Source: CAD feature listing. Evaluate the final solid. Frame: model axes, mm. Face numbers are marked on the shaded views. A direction names the side the tool comes from. Round coordinates to 2 decimals unless told otherwise and drop trailing zeros. Order: outer loops, then holes, each group sorted by start corner. A loop starts at its lowest first (then second) coordinate and runs counter-clockwise, first axis right, second up. Notation, with made-up numbers: (-28.75, 59.5) -> (21.25, 59.5) arc R32 cw to (21.25, 90.5) -> close; hole circle Ø9 at (61.5, -12). An arc over 180 degrees is marked (long way). Write item = value, one per line. Start each with the question number.
(1) Cut plane C-C on z = 11. Return the cut outline in (x, y), then the cut area to 3 significant figures.
(2) Cut plane D-D on x = -8. Return the cut outline in (y, z) (3 decimals), then the cut area to 3 significant figures.
(3) Cut plane A-A on z = 1.5. Return the cut outline in (x, y), then the cut area to 3 significant figures.
(4) Reachability of the marked faces 4, 5 and 6 from +Z, -Z, +X, -X, +Y, -Y: full face, straight path, thin tool, end or side. Return the list, or none.
(5) Contact query for flat-ended pins moving along their axis: pin 1 Ø5 at (y, z) = (1.5, 11) entering from +X; pin 2 Ø1.9 at (y, z) = (8, 21) entering from -X; pin 3 Ø10 at (x, y) = (-2, 6) entering from +Z (3 decimals); pin 4 Ø7 at (y, z) = (8, 19.6) entering from -X. Output: stop coordinate, or through.
(6) Ray query, line 1 (Y direction, x = 11.7, z = 19.6); line 2 (Y direction, x = 7, z = 19.25); line 3 (Z direction, x = 9, y = -1.75) (3 decimals). Return the intervals inside material, ascending.
(7) Draft query along X for the marked faces 1, 2 and 3. Return one class per face: released by +X, released by -X, zero draft, split by the parting line, or undercut.
(8) Cut plane B-B on y = 9.75. Return the cut outline in (x, z) (3 decimals).
from build123d import *

# Parameters (mm, degrees)
BOSS_EXTRUDE1_DEPTH   = 11.5
SKETCH3_R             = 2.4
CUT_EXTRUDE1_DEPTH    = 38.4
SKETCH3_3_R           = 3.1
SKETCH3_3_R_2         = 2.4
CUT_EXTRUDE2_DEPTH    = 0.8
FILLET1_R             = 3.6
F_8_CLEARANCE_HOLE1_D = 4.4958


with BuildPart() as part:
    # Sketch2 → Boss-Extrude1 (new body, symmetric)
    with BuildSketch(Plane(origin=(0, 0, 0), x_dir=(1, 0, 0), z_dir=(0, 1, 0))):
        Polygon((4, -3.175), (4, -19.599999916), (4, -23.199999916), (12, -23.199999916), (12, -19.599999916), (12, -3.175), (25.4, -3.175), (25.4, 3.175), (-25.4, 3.175), (-25.4, -3.175), align=None)
    extrude(amount=BOSS_EXTRUDE1_DEPTH, both=True)

    # Sketch3 → Cut-Extrude1 (cut, through all)
    with BuildSketch(Plane(origin=(12, 0, 0), x_dir=(0, 0, -1), z_dir=(1, 0, 0))):
        with Locations((-19.599999916, 8)):
            Circle(SKETCH3_R)
        with BuildLine():
            ThreePointArc((-17.337258216, 0.73137085), (-17.232272581, 0), (-17.337258216, -0.73137085))
            Line((-17.337258216, -0.73137085), (-18.799999916, -0.73137085))
            Line((-18.799999916, -0.73137085), (-18.799999916, -2.19411255))
            ThreePointArc((-18.799999916, -2.19411255), (-19.599999916, -2.320249175), (-20.399999916, -2.19411255))
            Line((-20.399999916, -2.19411255), (-20.399999916, -0.73137085))
            Line((-20.399999916, -0.73137085), (-21.862741616, -0.73137085))
            ThreePointArc((-21.862741616, -0.73137085), (-21.967727251, 0), (-21.862741616, 0.73137085))
            Line((-21.862741616, 0.73137085), (-20.399999916, 0.73137085))
            Line((-20.399999916, 0.73137085), (-20.399999916, 2.19411255))
            ThreePointArc((-20.399999916, 2.19411255), (-19.599999916, 2.320249175), (-18.799999916, 2.19411255))
            Line((-18.799999916, 2.19411255), (-18.799999916, 0.73137085))
            Line((-18.799999916, 0.73137085), (-17.337258216, 0.73137085))
        make_face()
        with Locations((-19.599999916, -8)):
            Circle(SKETCH3_R)
    extrude(amount=-CUT_EXTRUDE1_DEPTH, mode=Mode.SUBTRACT)

    # Sketch3_3 → Cut-Extrude2 (cut)
    with BuildSketch(Plane(origin=(12, 0, 0), x_dir=(0, 0, -1), z_dir=(1, 0, 0))):
        with Locations((-19.599999916, 8)):
            Circle(SKETCH3_3_R)
        with Locations((-19.599999916, 8)):
            Circle(SKETCH3_3_R_2, mode=Mode.SUBTRACT)
        with Locations((-19.599999916, -8)):
            Circle(SKETCH3_3_R)
        with Locations((-19.599999916, -8)):
            Circle(SKETCH3_3_R_2, mode=Mode.SUBTRACT)
    cut_extrude2 = extrude(amount=-CUT_EXTRUDE2_DEPTH, mode=Mode.SUBTRACT)

    # Mirror1: Cut-Extrude2 across plane
    add(cut_extrude2.mirror(Plane(origin=(8, 0, 0), x_dir=(0, 0, 1), z_dir=(1, 0, 0))), mode=Mode.SUBTRACT)

    # Fillet1
    fillet1_edges = [part.edges().sort_by_distance(p)[0] for p in [
        (8, -11.5, 23.199999916),
        (12, 0, 3.175),
        (4, 0, 3.175),
        (8, 11.5, 23.199999916),
    ]]
    fillet(fillet1_edges, radius=FILLET1_R)

    # 8 Clearance Hole1 (through all)
    with Locations(Plane.XY.offset(3.175)):
        with Locations((-20.6375, 6.7375), (-20.6375, -6.7375), (20.6375, -6.7375), (20.6375, 6.7375)):
            Hole(F_8_CLEARANCE_HOLE1_D / 2)


solid = part.part
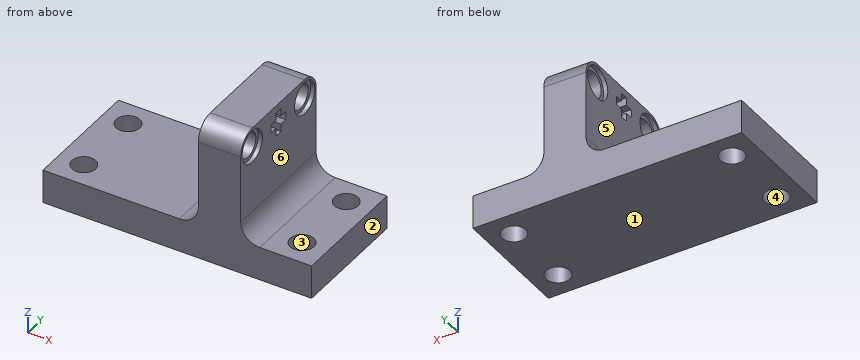
Evaluation:
q1.outline = (4, -11.5) -> (12, -11.5) -> (12, 11.5) -> (4, 11.5) -> close
q1.area = 184 mm^2
q2.outline = (-11.5, -3.175) -> (11.5, -3.175) -> (11.5, 3.175) -> (-11.5, 3.175) -> close
q2.area = 146 mm^2
q3.outline = (-25.4, -11.5) -> (25.4, -11.5) -> (25.4, 11.5) -> (-25.4, 11.5) -> close; hole circle Ø4.5 at (-20.64, -6.74); hole circle Ø4.5 at (-20.64, 6.74); hole circle Ø4.5 at (20.64, -6.74); hole circle Ø4.5 at (20.64, 6.74)
q3.area = 1,100 mm^2
q4.face_4 = +Z, -Z
q4.face_5 = +Z, -X, +Y, -Y
q4.face_6 = +Z, +X, +Y, -Y
q5.pin_1 = 12
q5.pin_2 = through
q5.pin_3 = 4.285
q5.pin_4 = 4
q6.line_1 = -11.5 to -11.1, -4.9 to -2.32, 2.32 to 4.9, 11.1 to 11.5
q6.line_2 = -11.5 to -10.37, -5.63 to -2.3, 2.3 to 5.63, 10.37 to 11.5
q6.line_3 = -3.175 to 18.8, 20.4 to 23.2
q7.face_1 = zero draft
q7.face_2 = released by +X
q7.face_3 = undercut
q8.outline = (-25.4, -3.175) -> (25.4, -3.175) -> (25.4, 3.175) -> (15.6, 3.175) arc R3.6 cw to (12, 6.775) -> (12, 17.041) -> (11.2, 17.041) -> (11.2, 17.958) -> (4.8, 17.958) -> (4.8, 17.041) -> (4, 17.041) -> (4, 6.775) arc R3.6 cw to (0.4, 3.175) -> (-25.4, 3.175) -> close; (4, 22.159) -> (4.8, 22.159) -> (4.8, 21.242) -> (11.2, 21.242) -> (11.2, 22.159) -> (12, 22.159) -> (12, 22.688) -> (4, 22.688) -> close
